```python
from build123d import *

# Parameters (mm, degrees)
SKETCH1_R               = 80.518
SKETCH1_R_2             = 67.818
INNER_CYLINDER_DEPTH    = 19.05
SKETCH2_R               = 104.775
SKETCH2_R_2             = 67.818
FLANGE_DEPTH            = 6.35
SKETCH4_R               = 81.407
SKETCH4_R_2             = 74.295
GROOVE_DEPTH            = 3.9878
SKETCH5_R               = 2.5527
SCREW_HOLES_DEPTH       = 6.35
CIRPATTERN1_COUNT       = 12
CUT_EXTRUDE1_DEPTH      = 3.6068
CUT_EXTRUDE1_DEPTH_BACK = 3.6068
SKETCH7_R               = 80.518
SKETCH7_R_2             = 76.1746


with BuildPart() as part:
    # Sketch1 → Inner Cylinder (new body)
    with BuildSketch(Plane(origin=(0, 0, 0), x_dir=(1, 0, 0), z_dir=(0, 1, 0))):
        with Locations(Location((0, 0, 0), (0, 0, 90))):
            Circle(SKETCH1_R)
        with Locations(Location((0, 0, 0), (0, 0, 90))):
            Circle(SKETCH1_R_2, mode=Mode.SUBTRACT)
    extrude(amount=INNER_CYLINDER_DEPTH)

    # Sketch2 → Flange (add)
    with BuildSketch(Plane(origin=(0, 19.05, 0), x_dir=(1, 0, 0), z_dir=(0, 1, 0))):
        with Locations(Location((0, 0, 0), (0, 0, 270))):
            Circle(SKETCH2_R)
        with Locations(Location((0, 0, 0), (0, 0, 90))):
            Circle(SKETCH2_R_2, mode=Mode.SUBTRACT)
    extrude(amount=FLANGE_DEPTH)

    # Sketch4 → Groove (cut)
    with BuildSketch(Plane(origin=(0, 25.4, 0), x_dir=(1, 0, 0), z_dir=(0, 1, 0))):
        with Locations(Location((0, 0, 0), (0, 0, 270))):
            Circle(SKETCH4_R)
        with Locations(Location((0, 0, 0), (0, 0, 270))):
            Circle(SKETCH4_R_2, mode=Mode.SUBTRACT)
    extrude(amount=-GROOVE_DEPTH, mode=Mode.SUBTRACT)

    # Sketch5 → Screw Holes (cut)
    with BuildSketch(Plane(origin=(0, 25.4, 0), x_dir=(1, 0, 0), z_dir=(0, 1, 0))):
        with Locations(Location((0, -97.25025, 0), (0, 0, 270))):
            Circle(SKETCH5_R)
    screw_holes = extrude(amount=-SCREW_HOLES_DEPTH, mode=Mode.SUBTRACT)

    # CirPattern1: Screw Holes ×12 about axis
    cirpattern1_axis = Axis((0, 0, 0), (0, 1, 0))
    for i in range(1, CIRPATTERN1_COUNT):
        add(screw_holes.rotate(cirpattern1_axis, i * 360 / CIRPATTERN1_COUNT), mode=Mode.SUBTRACT)

    # Sketch7 → Cut-Extrude1 (cut, two sides: drawn at the far end of the back side and taken through both)
    with BuildSketch(Plane(origin=(0, 9.525, 0), x_dir=(-1, 0, 0), z_dir=(0, -1, 0)).offset(-CUT_EXTRUDE1_DEPTH_BACK)):
        with Locations(Location((0, 0, 0), (0, 0, 90))):
            Circle(SKETCH7_R)
        with Locations(Location((0, 0, 0), (0, 0, 90))):
            Circle(SKETCH7_R_2, mode=Mode.SUBTRACT)
    extrude(amount=CUT_EXTRUDE1_DEPTH + CUT_EXTRUDE1_DEPTH_BACK, mode=Mode.SUBTRACT)


solid = part.part
```
Can you work these out from the model? Positions are in its coordinate system, mm. A direction names the side the tool comes from. Round coordinates to 2 decimals unless told otherwise and drop trailing zeros. Order: outer loops, then holes, each group sorted by start corner. A loop starts at its lowest first (then second) coordinate and runs counter-clockwise, first axis right, second up. Notation, with made-up numbers: (5.5, -16) -> (50.5, -16) arc R20 cw to (50.5, 13) -> close; hole circle Ø6 at (54, 24). An arc over 180 degrees is marked (long way). Return JSON: item names as keys, results as strings. Group by question number.
1. If we section it at C-C, the plane x = 0: Count the separate pieces of the cut face and the enclosed holes in it, then the cut area to 3 significant figures.
2. Will these pins go through, and if not, where does the flat tip stop? pin 1 (4.5 mm diameter, centred on x = 97.25, z = 0, fed in from -Y); pin 2 (5 mm diameter, centred on x = 49.5, z = 67.5, fed in from -Y); pin 3 (2 mm diameter, centred on x = -58.5, y = 22.5, fed in from -Z); pin 4 (10 mm diameter, centred on y = 12, z = 41, fed in from +X).
3. I need wall thicknesses on line 1 (X direction, y = 21.5, z = 15.5); line 2 (Z direction, x = -1, y = 6.5); line 3 (Y direction, x = -38.5, z = 91). Which ranges of each line are inside material? Lowest first, please. Write a range as [from, to].
4. We'd pull the mould along X, two halves only. Please class faces 4 (the face through (-85.774, 22.269, -50.651)), 5 (the face through (0.1, 22.3, 94.7)), 6 (the face through (-102.283, 22.181, -22.713)), 7 (the face through (-66, 25.4, -17)): released by +X, released by -X, zero draft, split by the parting line, or undercut.
5. If we section it at A-A, the plane x = -27.5: Write out the boundary of the cut face in (y, z).
6. Which directions (+Z, -Z, +X, -X, +Y, -Y) give clear straight access to the entire face, cutting with the end or side of a thin tool? Please do faces 1 (the face through (-50.651, 22.269, 85.774)), 2 (the face through (22.881, 9.575, -72.657)), 3 (the face through (-62, 19.05, 54)).
7. If we section it at B-B, the plane z = -9: Write out the boundary of the cut face in (x, y).
Output values:
{
 "1": {"separate pieces": "4", "enclosed holes": "0", "area": "769 mm²"},
 "2": {"pin 1": "through", "pin 2": "y = 19.05", "pin 3": "z = -87.59", "pin 4": "x = 71.96"},
 "3": {"line 1": "[-103.62, -79.92], [-72.66, -66.02], [66.02, 72.66], [79.92, 103.62]", "line 2": "[-76.17, -67.81], [67.81, 76.17]", "line 3": "[19.05, 25.4]"},
 "4": {"face 4": "undercut", "face 5": "undercut", "face 6": "split by the parting line", "face 7": "zero draft"},
 "5": {"outline": "(0, -75.68) -> (5.92, -75.68) -> (5.92, -71.04) -> (13.13, -71.04) -> (13.13, -75.68) -> (19.05, -75.68) -> (19.05, -101.1) -> (25.4, -101.1) -> (25.4, -76.62) -> (21.41, -76.62) -> (21.41, -69.02) -> (25.4, -69.02) -> (25.4, -61.99) -> (0, -61.99) -> close; (0, 61.99) -> (25.4, 61.99) -> (25.4, 69.02) -> (21.41, 69.02) -> (21.41, 76.62) -> (25.4, 76.62) -> (25.4, 101.1) -> (19.05, 101.1) -> (19.05, 75.68) -> (13.13, 75.68) -> (13.13, 71.04) -> (5.92, 71.04) -> (5.92, 75.68) -> (0, 75.68) -> close"},
 "6": {"face 1": "+Y, -Y", "face 2": "none", "face 3": "-Y"},
 "7": {"outline": "(-104.39, 19.05) -> (-80.01, 19.05) -> (-80.01, 13.13) -> (-75.64, 13.13) -> (-75.64, 5.92) -> (-80.01, 5.92) -> (-80.01, 0) -> (-67.22, 0) -> (-67.22, 25.4) -> (-73.75, 25.4) -> (-73.75, 21.41) -> (-80.91, 21.41) -> (-80.91, 25.4) -> (-104.39, 25.4) -> close; (67.22, 0) -> (80.01, 0) -> (80.01, 5.92) -> (75.64, 5.92) -> (75.64, 13.13) -> (80.01, 13.13) -> (80.01, 19.05) -> (104.39, 19.05) -> (104.39, 25.4) -> (80.91, 25.4) -> (80.91, 21.41) -> (73.75, 21.41) -> (73.75, 25.4) -> (67.22, 25.4) -> close"}
}
